Source: three-view drawing plus pictorial views. Frame: mm from the lowest corner of the part. A direction names the side the tool comes from. Round coordinates to 2 decimals unless told otherwise and drop trailing zeros. Loops run counter-clockwise (first coordinate to the right, second up) from the corner with the lowest first, then second, coordinate; pieces in that order, holes last. Notation, with made-up numbers: M -26.5,7 L 17.5,7 A26 ccw 17.5,34 Z; hole C 22.5,42.25 d3. An arc over 180 degrees is marked long. Answer as a JSON object with one key per item and string values.
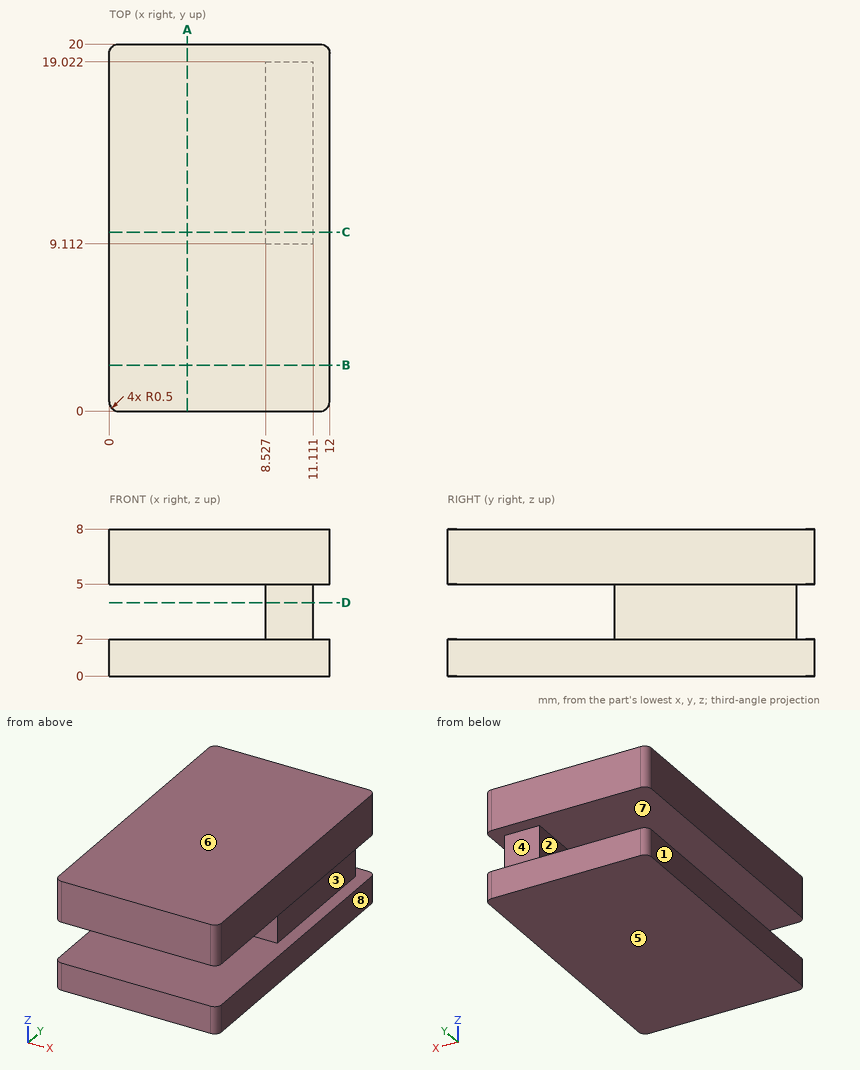
1) Cut plane A-A on x = 4.25. Return the cut outline in (y, z).
Geometry results:
{"outline": "M 0,0 L 20,0 L 20,2 L 0,2 Z; M 0,5 L 20,5 L 20,8 L 0,8 Z"}
2) Pull-direction query (Z, two-part tool) for the marked faces 5, 6, 7 and 8; classes: +Z half, -Z half, draft (parallel to the pull), parting line (faces both ways), or undercut.
Geometry results:
{"face 5": "-Z half", "face 6": "+Z half", "face 7": "undercut", "face 8": "draft"}
3) Line query: probe 1 along Z at (x, y) = (8.25, 5.25); probe 2 along Y at (x, z) = (10.5, 4.5); probe 3 along X at (y, z) = (13.75, 2.25). Output: solid intervals per line, ascending.
Geometry results:
{"probe 1": "0 to 2, 5 to 8", "probe 2": "9.11 to 19.02", "probe 3": "8.53 to 11.11"}
4) Set-up query: the marked faces 1, 2, 3 and 4. Return all of +Z, -Z, +X, -X, +Y, -Y with unobstructed straight access to the full face (end or side cutting, diameter ignored); none if empty.
Geometry results:
{"face 1": "+Z, -Z, -X, +Y, -Y", "face 2": "-X, +Y, -Y", "face 3": "+X, +Y, -Y", "face 4": "+X, -X, +Y"}
5) Cut plane B-B on y = 2.5. Return the cut outline in (x, z).
Geometry results:
{"outline": "M 0,0 L 12,0 L 12,2 L 0,2 Z; M 0,5 L 12,5 L 12,8 L 0,8 Z"}
6) Cut plane C-C on y = 9.75. Return the cut outline in (x, z).
Geometry results:
{"outline": "M 0,0 L 12,0 L 12,2 L 11.11,2 L 11.11,5 L 12,5 L 12,8 L 0,8 L 0,5 L 8.53,5 L 8.53,2 L 0,2 Z"}
7) Cut plane D-D on z = 4. Return the cut outline in (x, y), and give its area (3 significant figures).
Geometry results:
{"outline": "M 8.53,9.11 L 11.11,9.11 L 11.11,19.02 L 8.53,19.02 Z", "area": "25.6 mm2"}
8) First-contact query: pin 1 (1.5 mm diameter, centred on y = 16.5, z = 3, fed in from +X); pin 2 (0.8 mm diameter, centred on x = 9, z = 4, fed in from +Y); pin 3 (1.5 mm diameter, centred on y = 12, z = 3.5, fed in from -X). Flat tips, straight axial feed; report the tip coordinate or a pass-through.
Geometry results:
{"pin 1": "x = 11.11", "pin 2": "y = 19.02", "pin 3": "x = 8.53"}
